Work out the finished part from the listing and answer in its coordinate system (mm). A direction names the side the tool comes from. Give positions to 0.01 mm unless a question says otherwise; leave off trailing zeros. Order: outer loops, then holes, each group sorted by start corner. A loop starts at its lowest first (then second) coordinate and runs counter-clockwise, first axis right, second up.
```python
from build123d import *

# Parameters (mm, degrees)
SKETCH002_R  = 3.1
PAD001_DEPTH = 10
PAD_DEPTH    = 39
SKETCH001_R  = 37
POCKET_DEPTH = 37


with BuildPart() as pad001:
    # Sketch002 → Pad001 (new body)
    with BuildSketch(Plane.YZ.offset(29)):
        with Locations((0, 30)):
            Circle(SKETCH002_R)
        with Locations((0, 15)):
            Circle(SKETCH002_R)
    extrude(amount=PAD001_DEPTH)


with BuildPart() as cut:
    # Sketch → Pad (new body)
    with BuildSketch(Plane.XY):
        with BuildLine():
            ThreePointArc((37.696154, 10), (-39, 0), (37.696154, -10))
            Line((39.696154, -10), (37.696154, -10))
            Line((39.696154, 10), (39.696154, -10))
            Line((37.696154, 10), (39.696154, 10))
        make_face()
    extrude(amount=PAD_DEPTH)

    # Sketch001 → Pocket (cut)
    with BuildSketch(Plane.XY.offset(39)):
        Circle(SKETCH001_R)
    extrude(amount=-POCKET_DEPTH, mode=Mode.SUBTRACT)

    # Cut: cut Pad001
    add(pad001.part, mode=Mode.SUBTRACT)


solid = cut.part
```
1. The part is cut by section C-C (x = 0). Write down the section's boundary in (y, z), then the cut area to 3 significant figures.
Findings below:
outline: (-39, 0) - (39, 0) - (39, 39) - (37, 39) - (37, 2) - (-37, 2) - (-37, 39) - (-39, 39) - close
area: 304 mm2
2. The part is cut by section B-B (y = 0). Write down the section's boundary in (x, z), then the cut area to 3 significant figures.
Findings below:
outline: (-39, 0) - (39.7, 0) - (39.7, 39) - (37, 39) - (37, 33.1) - (39, 33.1) - (39, 26.9) - (37, 26.9) - (37, 18.1) - (39, 18.1) - (39, 11.9) - (37, 11.9) - (37, 2) - (-37, 2) - (-37, 39) - (-39, 39) - close
area: 306 mm2
3. Straight lines are drawn through the part: probe 1 along Z at (x, y) = (38.4, 0); probe 2 along Y at (x, z) = (38, 30); probe 3 along Y at (x, z) = (0, 24). For each, find the intervals that lie inside material, in ascending order.
Findings below:
probe 1: z = 0 to 11.9, 18.1 to 26.9, 33.1 to 39
probe 2: y = -10 to -3.1, 3.1 to 10
probe 3: y = -39 to -37, 37 to 39
4. Given P1, Ø4, axis at y = -23.5, z = 20, coming from the +X side; P2, Ø5, axis at y = -11.5, z = 19.5, coming from the +X side; P3, Ø3, axis at x = 10, y = -6, coming from the +Z side; P4, Ø5, axis at y = 0, z = 15, coming from the -X side, each flat-ended and moving along its own axis, determine where each tip first touches the part or whether it passes through.
Findings below:
P1: stops at x = 32.54
P2: stops at x = 39.7
P3: stops at z = 2
P4: stops at x = -39
5. The part is cut by section D-D (z = 4). Write down the section's boundary in (x, y).
Findings below:
outline: (37.7, -10) - (39.7, -10) - (39.7, 10) - (37.7, 10) arc R39 ccw (long way) to start; hole circle Ø74 at (0, 0)
6. Which of the six approach directions +Z, -Z, +X, -X, +Y, -Y give full straight-line access (tool end or side, diameter ignored) to faces 5 (the face through (39, -10, 19)), 6 (the face through (39, 0, 15)), 7 (the face through (-1, 1, 2))?
Findings below:
face 5: +Z, -Z, +X, -Y
face 6: none
face 7: +Z
7. The mould has two halves that part along Y. Classify faces 1 (the face through (-8.02, -36.12, 20.76)), 2 (the face through (0, 1, 0)), 3 (the face through (39, 10, 19)), 4 (the face through (37.92, 2.957, 30.931)): pulls with the +Y half, pulls with the -Y half, needs draft (parallel to the pull), parting line crosses it, or undercut.
Findings below:
face 1: undercut
face 2: needs draft
face 3: pulls with the +Y half
face 4: undercut
8. The part is cut by section A-A (z = 30). Write down the section's boundary in (x, y), then the cut area to 3 significant figures.
Findings below:
outline: (37.7, -10) - (39.7, -10) - (39.7, 10) - (37.7, 10) arc R39 ccw (long way) to start; hole (36.87, -3.1) - (39, -3.1) - (39, 3.1) - (36.87, 3.1) arc R37 ccw (long way) to start
area: 487 mm2
